For this review, take the finished solid that the model builds, in its own axes (mm). Face numbers are marked on the shaded views. A direction names the side the tool comes from. Give positions to 0.01 mm unless a question says otherwise; leave off trailing zeros. Order: outer loops, then holes, each group sorted by start corner. A loop starts at its lowest first (then second) coordinate and runs counter-clockwise, first axis right, second up. Notation, with made-up numbers: M -13,86 L 45,86 A13 cw 45,105 Z; hole C 6.25,60.5 d7. An arc over 180 degrees is marked long. Answer as CSV lines item,"result". Start each with the question number.
1. For line 1 along Z through (x, y) = (1.5, 12); line 2 along Z through (x, y) = (1.5, 4.25); line 3 along Y through (x, z) = (0.5, -2) (3 decimals), list the stretches that pass through material, from the lowest coordinate up.
2. We need section C-C, the plane z = -19.5. Give the boundary of the cut face in (x, y).
3. We need section B-B, the plane y = 0. Give the boundary of the cut face in (x, z).
4. Mouldability with a two-part tool opening along Y and no side actions: class the marked faces 4, 5 and 6 as pulls with the +Y half, pulls with the -Y half, needs draft (parallel to the pull), parting line crosses it, or undercut.
5. We need section D-D, the plane y = 4.5. Give the boundary of the cut face in (x, z), and give its area (3 significant figures).
6. Clearance check with flat-ended pins moving along their axes: P1, Ø2, axis at x = 7, z = -12, coming from the +Y side (3 decimals); P2, Ø1.4, axis at x = 8, z = 12, coming from the +Y side; P3, Ø0.6, axis at y = 11.5, z = 9.5, coming from the +X side. State where each tip first meets the part, or that it passes through.
7. Machinability: for the marked faces 1, 2 and 3, which of the approach directions +Z, -Z, +X, -X, +Y, -Y give a long, thin tool a straight path to every point of the face, cutting with its end or side? Answer none if there is none.
8. We need section A-A, the plane x = 6. Give the boundary of the cut face in (y, z) (3 decimals).
from build123d import *

# Parameters (mm, degrees)
BOSS_EXTRUDE2_DEPTH = 12
SKETCH2_R           = 2
BOSS_EXTRUDE3_DEPTH = 1
SKETCH3_R           = 1.5
BOSS_EXTRUDE4_DEPTH = 9
CUT_EXTRUDE1_START  = -9
CUT_EXTRUDE1_DEPTH  = 9
SKETCH5_W           = 1
SKETCH5_H           = 5.504032185
CUT_EXTRUDE2_DEPTH  = 35.052899636
SKETCH6_W           = 1
SKETCH6_H           = 1.293248053
CUT_EXTRUDE3_DEPTH  = 32.913534796
SKETCH7_W           = 8.674818334
SKETCH7_H           = 4.580598429
CUT_EXTRUDE4_DEPTH  = 2


with BuildPart() as part:
    # Sketch1 → Boss-Extrude2 (new body)
    with BuildSketch(Plane(origin=(0, 0, 0), x_dir=(0, 0, -1), z_dir=(1, 0, 0))):
        Polygon((7.575967815, 4.965), (-6.46289635, 4.965), (-6.46289635, 8.187263597), (-4.840898274, 9.809261674), (-4.840898274, 14.205), (-7.55, 14.205), (-7.55, 12.920980416), (-13.054032185, 12.920980416), (-13.054032185, 6.270822131), (-11.130968968, 6.270822131), (-9.825146836, 4.965), (-7.55, 4.965), (-7.55, -4.965), (7.55, -4.965), (16.375967815, -4.965), (16.375967815, 4.965), align=None)
    extrude(amount=BOSS_EXTRUDE2_DEPTH)

    # Sketch2 → Boss-Extrude3 (add)
    with BuildSketch(Plane(origin=(0, 0, -16.375967815), x_dir=(-1, 0, 0), z_dir=(0, 0, -1))):
        with Locations((-6, 0)):
            Circle(SKETCH2_R)
    extrude(amount=BOSS_EXTRUDE3_DEPTH)

    # Sketch3 → Boss-Extrude4 (add)
    with BuildSketch(Plane(origin=(0, 0, -17.375967815), x_dir=(-1, 0, 0), z_dir=(0, 0, -1))):
        with Locations((-6, 0)):
            Circle(SKETCH3_R)
    extrude(amount=BOSS_EXTRUDE4_DEPTH)

    # Sketch4 → Cut-Extrude1 (cut)
    with BuildSketch(Plane(origin=(0, 0, -26.375967815), x_dir=(-1, 0, 0), z_dir=(0, 0, -1)).offset(CUT_EXTRUDE1_START)):
        with BuildLine():
            Line((-6.839845518, -1.242843315), (-5.160154482, -1.242843315))
            ThreePointArc((-5.160154482, -1.242843315), (-6, -1.5), (-6.839845518, -1.242843315))
        make_face()
    extrude(amount=CUT_EXTRUDE1_DEPTH, mode=Mode.SUBTRACT)

    # Sketch5 → Cut-Extrude2 (cut, through all)
    with BuildSketch(Plane(origin=(0, 12.920980416, 0), x_dir=(1, 0, 0), z_dir=(0, 1, 0))):
        with Locations((11.5, -10.302016093)):
            Rectangle(SKETCH5_W, SKETCH5_H)
        with Locations((0.5, -10.302016093)):
            Rectangle(SKETCH5_W, SKETCH5_H)
    extrude(amount=-CUT_EXTRUDE2_DEPTH, mode=Mode.SUBTRACT)

    # Sketch6 → Cut-Extrude3 (cut, through all)
    with BuildSketch(Plane(origin=(11, 0, 0), x_dir=(0, 0, -1), z_dir=(1, 0, 0))):
        with Locations((-10.802016092, 12.27435639)):
            Rectangle(SKETCH6_W, SKETCH6_H)
    extrude(amount=-CUT_EXTRUDE3_DEPTH, mode=Mode.SUBTRACT)

    # Sketch7 → Cut-Extrude4 (cut)
    with BuildSketch(Plane(origin=(0, 12.920980416, 0), x_dir=(1, 0, 0), z_dir=(0, 1, 0))):
        with Locations((6, -10.302016093)):
            Rectangle(SKETCH7_W, SKETCH7_H)
    extrude(amount=-CUT_EXTRUDE4_DEPTH, mode=Mode.SUBTRACT)


solid = part.part
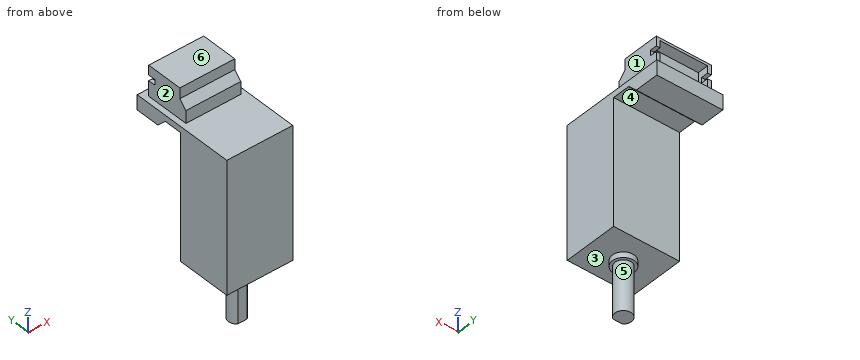
Result set:
1,line 1,"4.84 to 10.3, 11.3 to 13.05"
1,line 2,"-16.38 to 7.55"
1,line 3,"-4.965 to 4.965"
2,outline,"M 5.16,-1.24 L 6.84,-1.24 A1.5 ccw long Z"
3,outline,"M 0,-16.38 L 4,-16.38 L 4,-17.38 L 4.5,-17.38 L 4.5,-26.38 L 7.5,-26.38 L 7.5,-17.38 L 8,-17.38 L 8,-16.38 L 12,-16.38 L 12,7.55 L 0,7.55 Z"
4,face 4,"undercut"
4,face 5,"parting line crosses it"
4,face 6,"needs draft"
5,outline,"M 0,-16.38 L 12,-16.38 L 12,7.55 L 0,7.55 Z"
5,area,"287 mm2"
6,P1,"y = 4.965"
6,P2,"y = 12.92"
6,P3,"x = 11"
7,face 1,"+Z, +X, +Y, -Y"
7,face 2,"+Z, -X, +Y, -Y"
7,face 3,"-Z"
8,outline,"M -4.965,-16.376 L -2,-16.376 L -2,-17.376 L -1.243,-17.376 L -1.243,-26.376 L 1.5,-26.376 L 1.5,-17.376 L 2,-17.376 L 2,-16.376 L 4.965,-16.376 L 4.965,6.463 L 8.187,6.463 L 9.809,4.841 L 14.205,4.841 L 14.205,7.55 L 12.921,7.55 L 12.921,8.012 L 10.921,8.012 L 10.921,12.592 L 12.921,12.592 L 12.921,13.054 L 6.271,13.054 L 6.271,11.131 L 4.965,9.825 L 4.965,7.55 L -4.965,7.55 Z"
